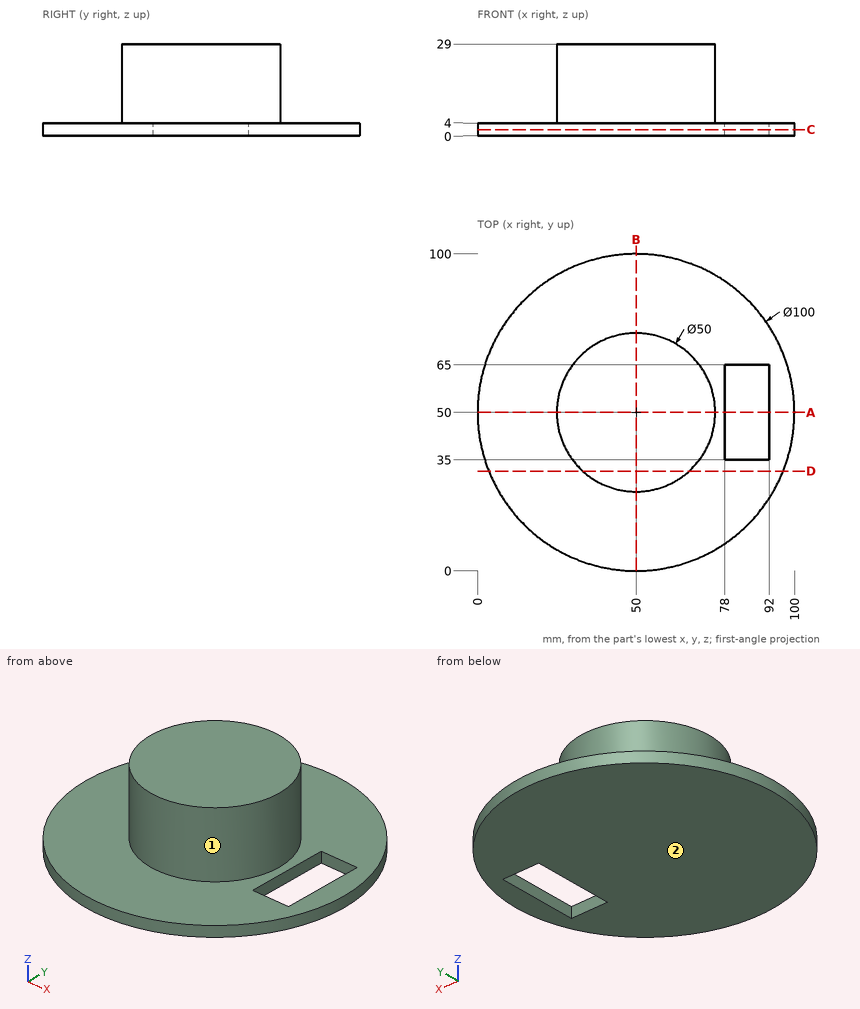
Part print with two shaded views. Sizes in mm from the minimum x, y, z corner. A direction names the side the tool comes from. Round coordinates to 2 decimals unless told otherwise and drop trailing zeros. Order: outer loops, then holes, each group sorted by start corner. A loop starts at its lowest first (then second) coordinate and runs counter-clockwise, first axis right, second up. Notation, with made-up numbers: (-4.75, 57.5) -> (46.25, 57.5) arc R30 cw to (46.25, 85.5) -> close; hole circle Ø7 at (11, -4). An arc over 180 degrees is marked (long way). Use one line per item in the form item = value.
Item 1: Cut at A-A, the plane y = 50. Write the cut outline in (x, z).
Returned:
outline = (0, 0) -> (78, 0) -> (78, 4) -> (75, 4) -> (75, 29) -> (25, 29) -> (25, 4) -> (0, 4) -> close; (92, 0) -> (100, 0) -> (100, 4) -> (92, 4) -> close
Item 2: Cut at D-D, the plane y = 31.5. Write the cut outline in (x, z), and give its area (3 significant figures).
Returned:
outline = (3.55, 0) -> (96.45, 0) -> (96.45, 4) -> (66.82, 4) -> (66.82, 29) -> (33.18, 29) -> (33.18, 4) -> (3.55, 4) -> close
area = 1,210 mm^2
Item 3: Tool access for the marked faces 1 and 2: list every direction of +Z, -Z, +X, -X, +Y, -Y with a clear straight run to the whole face (end or side of a thin tool).
Returned:
face_1 = +Z
face_2 = -Z, +X, -X, +Y, -Y
Item 4: Cut at B-B, the plane x = 50. Write the cut outline in (y, z).
Returned:
outline = (0, 0) -> (100, 0) -> (100, 4) -> (75, 4) -> (75, 29) -> (25, 29) -> (25, 4) -> (0, 4) -> close
Item 5: Drill centre lines: line 1 (Z direction, x = 65, y = 20); line 2 (Y direction, x = 49, z = 24); line 3 (Y direction, x = 39, z = 11.5). Where is each one in solid material? Low to high.
Returned:
line_1 = 0 to 4
line_2 = 25.02 to 74.98
line_3 = 27.55 to 72.45
Item 6: Flat gauge pins, fed straight in: pin 1 Ø1.2 at (x, z) = (84, 1.5) entering from +Y; pin 2 Ø10 at (x, z) = (49, 12) entering from -Y; pin 3 Ø1.2 at (x, z) = (82, 2) entering from -Y. Where does each tip first touch, or does it go through?
Returned:
pin_1 = 87.21
pin_2 = 25
pin_3 = 11.09
Item 7: Cut at C-C, the plane z = 2. Write the cut outline in (x, y).
Returned:
outline = circle Ø100 at (50, 50); hole (78, 35) -> (92, 35) -> (92, 65) -> (78, 65) -> close
